The model under review builds one solid part; all positions refer to its coordinate system, in mm. Give positions to 0.01 mm unless a question says otherwise; leave off trailing zeros. Order: outer loops, then holes, each group sorted by start corner. A loop starts at its lowest first (then second) coordinate and runs counter-clockwise, first axis right, second up. Notation, with made-up numbers: M 12,70.25 L 42,70.25 A25 cw 42,88.25 Z; hole C -25.5,-22 d5. An arc over 180 degrees is marked long. One line per question, with ' | ' between items. Start each with the question number.
1. Wall thickness on L1, parallel to Y at x = 1.05, z = 1350; L2, parallel to Y at x = 29.7, z = 718.5; L3, parallel to X at y = 15, z = 491.5: over which ranges is each line inside the solid? List them lowest first.
2. We need section A-A on y = 41. Write out the cut boundary in (x, z).
3. Insertion check: P1, Ø10, axis at x = 11.5, y = 10.5, coming from the +Z side; P2, Ø5.5, axis at y = 25, z = 700, coming from the +X side. Each pin has a flat end and moves straight along its axis. Give the tip position at first contact, or say it passes through.
4. We need section B-B on x = 21. Write out the cut boundary in (y, z), then the cut area to 3 significant figures.
5. We need section C-C on z = 1152.5. Write out the cut boundary in (x, y), then the cut area to 3 significant figures.
```python
from build123d import *

# Parameters (mm, degrees)
ESBO_O1_W                   = 30
ESBO_O1_H                   = 50
ESBO_O1_W_2                 = 27
ESBO_O1_H_2                 = 47
RESSALTO_EXTRUS_O1_DEPTH    = 1400
FURO_COM_FOLGA_DE_M52_D     = 5.5
FURO_COM_FOLGA_DE_M81_D     = 9
FURO_COM_FOLGA_DE_M84_D     = 9
FURO_COM_FOLGA_DE_M84_DEPTH = 1.5


with BuildPart() as part:
    # Esboço1 → Ressalto-extrusão1 (new body)
    with BuildSketch(Plane.XY):
        with Locations((15, 25)):
            Rectangle(ESBO_O1_W, ESBO_O1_H)
        with Locations((15, 25)):
            Rectangle(ESBO_O1_W_2, ESBO_O1_H_2, mode=Mode.SUBTRACT)
    extrude(amount=RESSALTO_EXTRUS_O1_DEPTH)

    # Furo com folga de M52 (through all)
    with Locations(Plane(origin=(30, 0, 0), x_dir=(0, 0, -1), z_dir=(1, 0, 0))):
        with Locations((-1368.5, 25), (-1331.5, 25), (-68.5, 25), (-31.5, 25), (-718.5, 25), (-681.5, 25)):
            Hole(FURO_COM_FOLGA_DE_M52_D / 2)

    # Furo com folga de M81 (through all)
    with Locations(Plane(origin=(30, 0, 0), x_dir=(0, 0, -1), z_dir=(1, 0, 0))):
        with Locations((-1350, 25), (-50, 25)):
            Hole(FURO_COM_FOLGA_DE_M81_D / 2)

    # Furo com folga de M84
    with Locations(Plane(origin=(30, 0, 0), x_dir=(0, 0, -1), z_dir=(1, 0, 0))):
        with Locations((-700, 25)):
            Hole(FURO_COM_FOLGA_DE_M84_D / 2, depth=FURO_COM_FOLGA_DE_M84_DEPTH)


solid = part.part
```
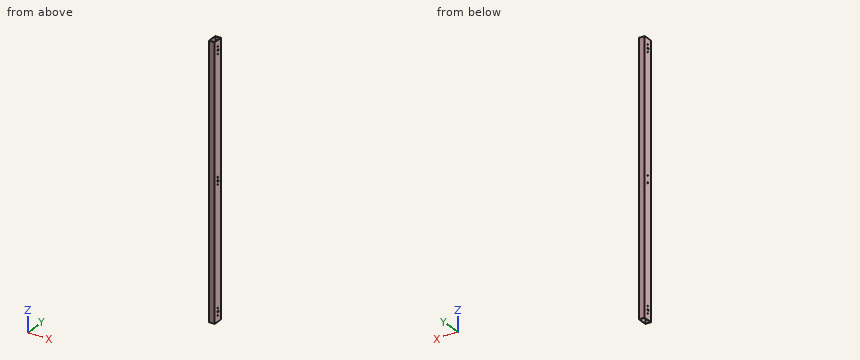
Entries:
1) L1: y = 0 to 20.5, 29.5 to 50 | L2: y = 0 to 22.25, 27.75 to 50 | L3: x = 0 to 1.5, 28.5 to 30
2) outline: M 0,0 L 1.5,0 L 1.5,1400 L 0,1400 Z; M 28.5,0 L 30,0 L 30,1400 L 28.5,1400 Z
3) P1: passes through | P2: stops at x = 1.5
4) outline: M 0,0 L 1.5,0 L 1.5,1400 L 0,1400 Z; M 48.5,0 L 50,0 L 50,1400 L 48.5,1400 Z | area: 4,200 mm^2
5) outline: M 0,0 L 30,0 L 30,50 L 0,50 Z; hole M 1.5,1.5 L 28.5,1.5 L 28.5,48.5 L 1.5,48.5 Z | area: 231 mm^2
